Read the model definition and answer for the solid it produces. Units are mm, in the model's axes. Face numbers are marked on the shaded views. A direction names the side the tool comes from. Coordinates: 2 decimals unless noted, no trailing zeros. Write each loop counter-clockwise with the first axis right and the second up, starting at its lowest first coordinate (ties: lowest second). Pieces come first, ordered by that corner, then holes.
Item 1: A tool of negligible diameter and unlimited length cuts with its end or side. For the marked faces 4, 5 and 6, from which of +Z, -Z, +X, -X, +Y, -Y can it reach the whole face along a straight path? Write none if from no direction.
Item 2: Each of these flat-tipped pins is pushed along its axis until it touches: P1, Ø0.9, axis at y = 26, z = -7, coming from the +X side; P2, Ø0.6, axis at x = -19.5, y = 29, coming from the +Z side. Where does it stop, or does it pass through?
Item 3: Determine the mould class of the marked faces 1, 2 and 3 for opening direction X: released by +X, released by -X, zero draft, split by the parting line, or undercut.
Item 4: Section D-D (z = -8.15) is taken. Give the vertices of the cut face in (x, y), then the cut area to 3 significant figures.
Item 5: Section A-A (y = 28.4) is taken. Give the vertices of the cut face in (x, z).
Item 6: Section B-B (x = -16) is taken. Give the vertices of the cut face in (y, z), then the cut area to 3 significant figures.
Item 7: Section C-C (y = 24.5) is taken. Give the vertices of the cut face in (x, z), then the cut area to 3 significant figures.
Item 8: Straight lines are drawn through the part: probe 1 along Y at (x, z) = (-16, -9.05); probe 2 along X at (y, z) = (25, -7.2); probe 3 along Y at (x, z) = (-14.25, -9.35). For each, find the intervals that lie inside material, in ascending order.
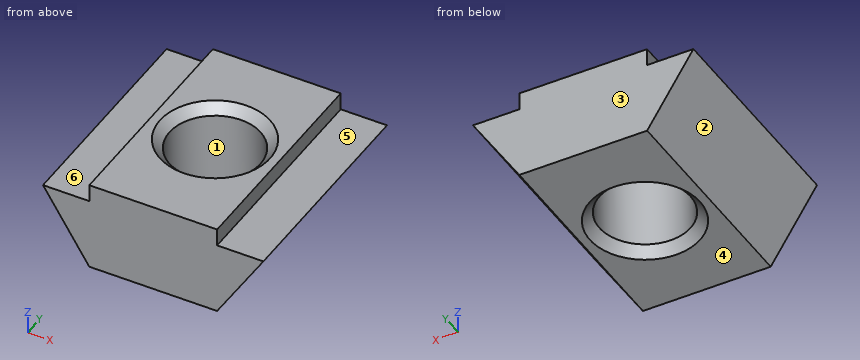
from build123d import *

# Parameters (mm, degrees)
EXTRUDE1_DEPTH = 10
SKETCH2_W      = 5.8
SKETCH2_H      = 10
EXTRUDE2_DEPTH = 0.8
HOLEWZD1_D     = 4.134
HOLEWZD1_DEPTH = 4.1
CHAMFER1_SIZE  = 0.433


with BuildPart() as part:
    # Sketch1 → Extrude1 (new body)
    with BuildSketch(Plane.XZ.offset(-23.4)):
        Polygon((-13.1, -10.8), (-11, -7.5), (-21, -7.5), (-18.9, -10.8), align=None)
    extrude(amount=-EXTRUDE1_DEPTH)

    # Sketch2 → Extrude2 (add)
    with BuildSketch(Plane.XY.offset(-7.5)):
        with Locations((-16, 28.4)):
            Rectangle(SKETCH2_W, SKETCH2_H)
    extrude(amount=EXTRUDE2_DEPTH)

    # HoleWzd1
    with Locations(Plane.XY.offset(-6.7)):
        with Locations((-16, 28.4)):
            Hole(HOLEWZD1_D / 2, depth=HOLEWZD1_DEPTH)

    # Chamfer1
    chamfer1_edges = [part.edges().sort_by_distance(p)[0] for p in [
        (-13.933, 28.4, -6.7),
        (-13.933, 28.4, -10.8),
    ]]
    chamfer(chamfer1_edges, length=CHAMFER1_SIZE)


solid = part.part
Established:
1. face 4: -Z, +X, -X, +Y, -Y
1. face 5: +Z, +X, +Y, -Y
1. face 6: +Z, -X, +Y, -Y
2. P1: stops at x = -13.1
2. P2: stops at z = -7.5
3. face 1: undercut
3. face 2: released by -X
3. face 3: zero draft
4. outline: (-20.59, 23.4) - (-11.41, 23.4) - (-11.41, 33.4) - (-20.59, 33.4) - close; hole circle Ø4.13 at (-16, 28.4)
4. area: 78.3 mm2
5. outline: (-21, -7.5) - (-18.9, -10.8) - (-18.5, -10.8) - (-18.07, -10.37) - (-18.07, -7.13) - (-18.5, -6.7) - (-18.9, -6.7) - (-18.9, -7.5) - close; (-13.93, -10.37) - (-13.5, -10.8) - (-13.1, -10.8) - (-11, -7.5) - (-13.1, -7.5) - (-13.1, -6.7) - (-13.5, -6.7) - (-13.93, -7.13) - close
6. outline: (23.4, -10.8) - (25.9, -10.8) - (26.33, -10.37) - (26.33, -7.13) - (25.9, -6.7) - (23.4, -6.7) - close; (30.47, -10.37) - (30.9, -10.8) - (33.4, -10.8) - (33.4, -6.7) - (30.9, -6.7) - (30.47, -7.13) - close
6. area: 23.7 mm2
7. outline: (-21, -7.5) - (-18.9, -10.8) - (-13.1, -10.8) - (-11, -7.5) - (-13.1, -7.5) - (-13.1, -6.7) - (-18.9, -6.7) - (-18.9, -7.5) - close
7. area: 30.7 mm2
8. probe 1: y = 23.4 to 26.33, 30.47 to 33.4
8. probe 2: x = -18.9 to -13.1
8. probe 3: y = 23.4 to 27.3, 29.5 to 33.4
